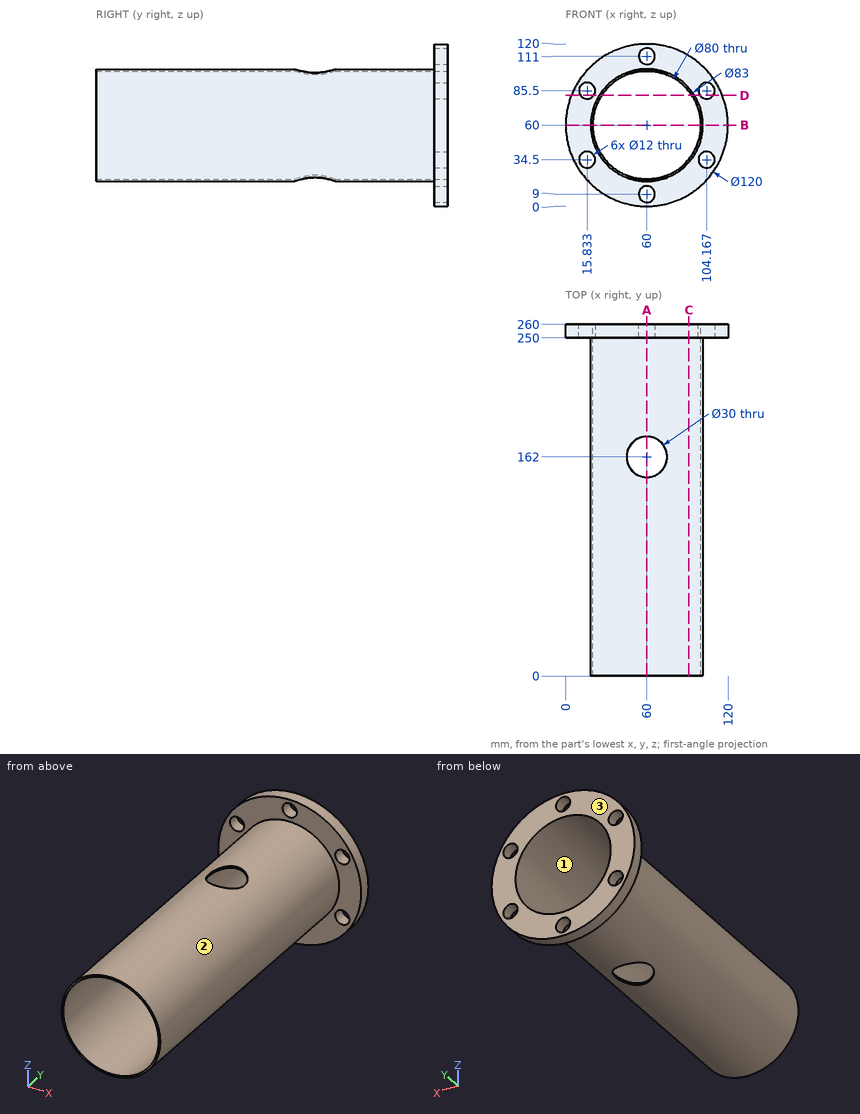
Check sheet for the drawn part. Datum: minimum x, y, z corner. Units: mm. Round coordinates to 2 decimals unless told otherwise and drop trailing zeros. Order: outer loops, then holes, each group sorted by start corner. A loop starts at its lowest first (then second) coordinate and runs counter-clockwise, first axis right, second up.
1) Section check C-C (x = 91). Record the boundary of the cut face in (y, z).
2) Section check D-D (z = 82). Record the boundary of the cut face in (x, y).
3) Mould release check, pull along Z, two halves, no side actions. Record for the marked faces 1, 2 and 3: +Z half, -Z half, draft (parallel to the pull), parting line (faces both ways), or undercut.
4) Section check A-A (x = 60). Record the boundary of the cut face in (y, z).
5) Section check B-B (z = 60). Record the boundary of the cut face in (x, y).
6) Scan lines: line 1 (Z direction, x = 60, y = 256); line 2 (Y direction, x = 60, z = 19); line 3 (X direction, y = 254, z = 85) (1 decimal). Record each from-to range of solid material in increasing order.
7) Go/stop test with flat-tipped pins: pin 1 Ø1 at (y, z) = (121.5, 67.5) entering from -X (1 decimal); pin 2 Ø3 at (y, z) = (118.5, 44.5) entering from +X; pin 3 Ø3 at (x, y) = (70.5, 172.5) entering from +Z. Record where each tip stops, or that it passes through.
Result:
1. outline: (0, 32.41) - (250, 32.41) - (250, 8.63) - (260, 8.63) - (260, 34.72) - (0, 34.72) - close; (0, 85.28) - (260, 85.28) - (260, 111.37) - (250, 111.37) - (250, 87.59) - (0, 87.59) - close
2. outline: (4.18, 250) - (10.96, 250) - (10.96, 260) - (4.18, 260) - close; (20.71, 250) - (24.81, 250) - (24.81, 0) - (26.59, 0) - (26.59, 260) - (20.71, 260) - close; (93.41, 0) - (95.19, 0) - (95.19, 250) - (99.29, 250) - (99.29, 260) - (93.41, 260) - close; (109.04, 250) - (115.82, 250) - (115.82, 260) - (109.04, 260) - close
3. face 1: undercut
3. face 2: parting line
3. face 3: draft
4. outline: (0, 18.5) - (147, 18.5) - (147, 20) - (0, 20) - close; (0, 100) - (147, 100) - (147, 101.5) - (0, 101.5) - close; (177, 18.5) - (250, 18.5) - (250, 15) - (260, 15) - (260, 20) - (177, 20) - close; (177, 100) - (260, 100) - (260, 105) - (250, 105) - (250, 101.5) - (177, 101.5) - close; (250, 0) - (260, 0) - (260, 3) - (250, 3) - close; (250, 117) - (260, 117) - (260, 120) - (250, 120) - close
5. outline: (0, 250) - (18.5, 250) - (18.5, 0) - (20, 0) - (20, 260) - (0, 260) - close; (100, 0) - (101.5, 0) - (101.5, 250) - (120, 250) - (120, 260) - (100, 260) - close
6. line 1: z = 0 to 3, 15 to 20, 100 to 105, 117 to 120
6. line 2: y = 0 to 147, 177 to 260
6. line 3: x = 5.5 to 9.9, 21.8 to 28.8, 91.2 to 98.2, 110.1 to 114.5
7. pin 1: stops at x = 19.1
7. pin 2: stops at x = 99.07
7. pin 3: stops at z = 100.4
